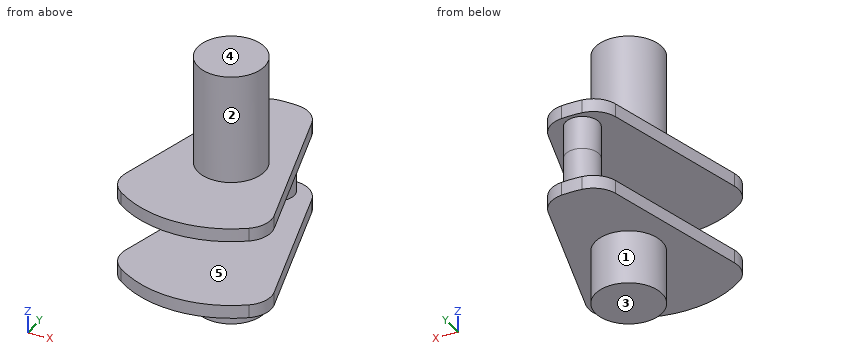
```python
from build123d import *

# Parameters (mm, degrees)
BOSS_EXTRUDE1_DEPTH = 20.32
SKETCH2_R           = 25.4
BOSS_EXTRUDE2_DEPTH = 50.8
SKETCH4_R           = 50.8
BOSS_EXTRUDE3_DEPTH = 82.804
SKETCH5_R           = 50.8
BOSS_EXTRUDE4_DEPTH = 84.836
SKETCH6_W           = 2.54
SKETCH6_H           = 12.7
CUT_EXTRUDE1_DEPTH  = 2.54


with BuildPart() as part:
    # Sketch1 → Boss-Extrude1 (new body)
    with BuildSketch(Plane.XY):
        with BuildLine():
            Line((-50.872217321, 134.585225504), (-112.061443675, -90.240779366))
            ThreePointArc((-112.061443675, -90.240779366), (-111.162689162, -114.462461255), (-96.634871694, -133.864526939))
            ThreePointArc((-96.634871694, -133.864526939), (0, -165.1), (96.634871694, -133.864526939))
            ThreePointArc((96.634871694, -133.864526939), (111.162689162, -114.462461255), (112.061443675, -90.240779366))
            Line((112.061443675, -90.240779366), (50.872217321, 134.585225504))
            ThreePointArc((50.872217321, 134.585225504), (37.822210961, 155.010576595), (15.465489796, 164.374050949))
            ThreePointArc((15.465489796, 164.374050949), (0, 165.1), (-15.465489796, 164.374050949))
            ThreePointArc((-15.465489796, 164.374050949), (-37.822210961, 155.010576595), (-50.872217321, 134.585225504))
        make_face()
    extrude(amount=BOSS_EXTRUDE1_DEPTH)

    # Sketch2 → Boss-Extrude2 (add)
    with BuildSketch(Plane.XY.offset(20.32)):
        with Locations((0, 133.5786)):
            Circle(SKETCH2_R)
    extrude(amount=BOSS_EXTRUDE2_DEPTH)

    # Sketch4 → Boss-Extrude3 (add)
    with BuildSketch(Plane(origin=(0, 0, 0), x_dir=(-1, 0, 0), z_dir=(0, 0, -1))):
        with Locations(Location((0, 0, 0), (0, 0, 180))):
            Circle(SKETCH4_R)
    extrude(amount=BOSS_EXTRUDE3_DEPTH)

    # Mirror1: part across plane


with BuildPart() as part_1:
    add(part.part)
    add(part.part.mirror(Plane(origin=(0, 133.5786, 71.12), x_dir=(1, 0, 0), z_dir=(0, 0, 1))))

    # Sketch5 → Boss-Extrude4 (add)
    with BuildSketch(Plane.XY.offset(225.044)):
        Circle(SKETCH5_R)
    extrude(amount=BOSS_EXTRUDE4_DEPTH)

    # Sketch6 → Cut-Extrude1 (cut)
    with BuildSketch(Plane.XY.offset(142.24)):
        with Locations((1.27, 61.148656496)):
            Rectangle(SKETCH6_W, SKETCH6_H)
    extrude(amount=-CUT_EXTRUDE1_DEPTH, mode=Mode.SUBTRACT)


solid = part_1.part
```
The listing builds one solid part. Answer for the finished solid, in the listing's coordinates (mm). Face numbers are marked on the shaded views. A direction names the side the tool comes from. Coordinates: 2 decimals unless noted, no trailing zeros. Order: outer loops, then holes, each group sorted by start corner. A loop starts at its lowest first (then second) coordinate and runs counter-clockwise, first axis right, second up. Notation, with made-up numbers: M 38,51 L 64,51 A12 ccw 64,69 Z; hole C -40,0 d1. An arc over 180 degrees is marked long. Answer as a JSON object with one key per item and string values. Group by question number.
1. Determine the mould class of the marked faces 3, 4 and 5 for opening direction Z: released by +Z, released by -Z, zero draft, split by the parting line, or undercut.
2. Flat-ended cylindrical pins translate along their axes: P1, Ø10, axis at x = -51.5, z = -17.5, coming from the -Y side; P2, Ø4, axis at x = 51, y = -34, coming from the -Z side; P3, Ø2, axis at x = 1.5, z = 140.5, coming from the -Y side. Find the tip coordinate at first contact, or state that the pin passes through.
3. Section D-D on y = 0 is taken. Write down the section's boundary in (x, z).
4. Section A-A on y = -96 is taken. Write down the section's boundary in (x, z).
5. Section B-B on y = 38 is taken. Write down the section's boundary in (x, z).
6. A tool of negligible diameter and unlimited length cuts with its end or side. For the marked faces 1 and 2, from which of +Z, -Z, +X, -X, +Y, -Y can it reach the whole face along a straight path? Write none if from no direction.
7. Straight lines are drawn through the part: line 1 (Z direction, x = 57, y = -119); line 2 (Z direction, x = -1, y = -11); line 3 (Y direction, x = 15, z = 81). For each, find the intervals that lie inside material, in ascending order.
8. Section C-C on z = 191 is taken. Write down the section's boundary in (x, y), then the cut area to 3 significant figures.
Values follow:
{
 "1": {"face 3": "released by -Z", "face 4": "released by +Z", "face 5": "undercut"},
 "2": {"P1": "y = -20.45", "P2": "z = 0", "P3": "y = -165.1"},
 "3": {"outline": "M -87.5,0 L -50.8,0 L -50.8,-82.8 L 50.8,-82.8 L 50.8,0 L 87.5,0 L 87.5,20.32 L -87.5,20.32 Z; M -87.5,121.92 L 87.5,121.92 L 87.5,142.24 L 50.8,142.24 L 50.8,309.88 L -50.8,309.88 L -50.8,142.24 L -87.5,142.24 Z"},
 "4": {"outline": "M -113.19,0 L 113.19,0 L 113.19,20.32 L -113.19,20.32 Z; M -113.19,121.92 L 113.19,121.92 L 113.19,142.24 L -113.19,142.24 Z"},
 "5": {"outline": "M -77.16,0 L -33.71,0 L -33.71,-82.8 L 33.71,-82.8 L 33.71,0 L 77.16,0 L 77.16,20.32 L -77.16,20.32 Z; M -77.16,121.92 L 77.16,121.92 L 77.16,142.24 L 33.71,142.24 L 33.71,309.88 L -33.71,309.88 L -33.71,142.24 L -77.16,142.24 Z"},
 "6": {"face 1": "-Z", "face 2": "+Z"},
 "7": {"line 1": "0 to 20.32, 121.92 to 142.24", "line 2": "-82.8 to 20.32, 121.92 to 309.88", "line 3": "113.08 to 154.08"},
 "8": {"outline": "C 0,0 d101.6", "area": "8,110 mm2"}
}
